Source: three-view drawing plus pictorial views. Frame: mm from the lowest corner of the part. A direction names the side the tool comes from. Give positions to 0.01 mm unless a question says otherwise; leave off trailing zeros. Order: outer loops, then holes, each group sorted by start corner. A loop starts at its lowest first (then second) coordinate and runs counter-clockwise, first axis right, second up. Notation, with made-up numbers: (57.5, -23) - (69.5, -23) arc R25 ccw to (69.5, 9) - close; hole circle Ø8 at (-7, 36). An arc over 180 degrees is marked (long way). Answer in a Markdown table with one row per item. Add a question column.
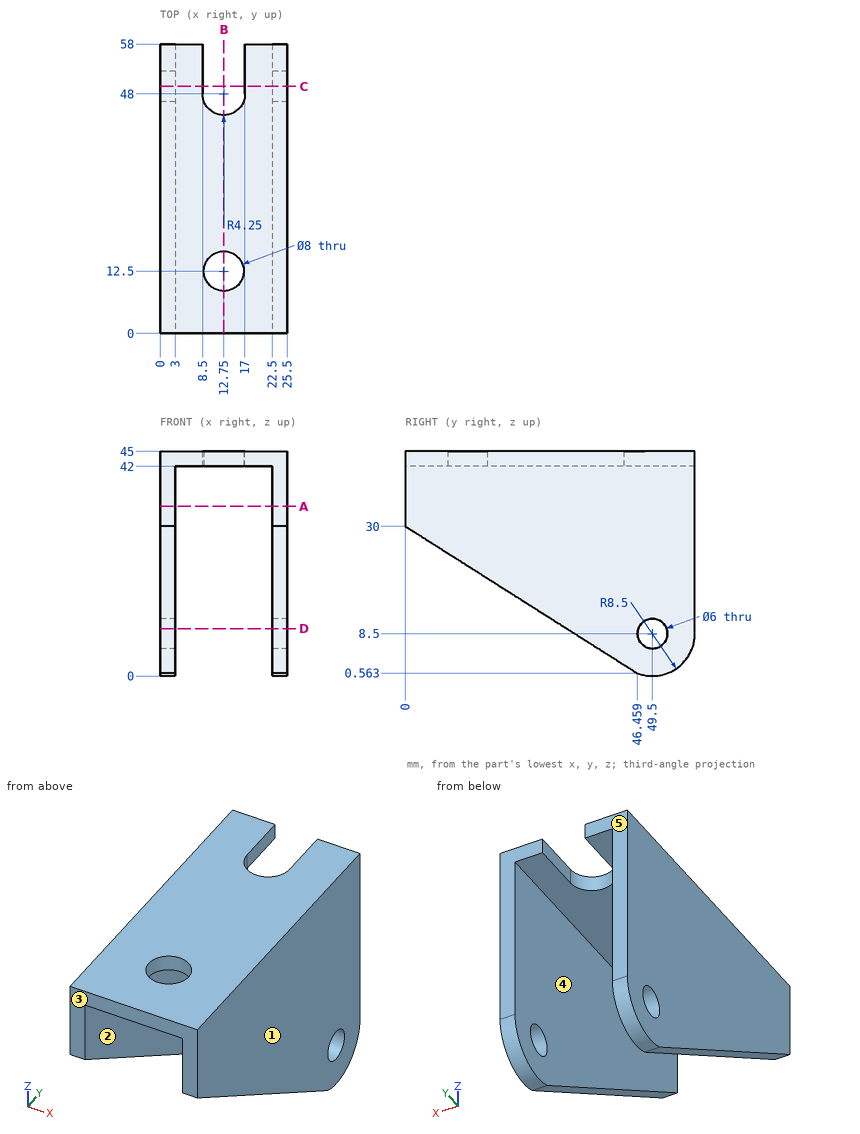
Q1. Pull-direction query (X, two-part tool) for the marked faces 1, 2 and 3; classes: +X half, -X half, draft (parallel to the pull), parting line (faces both ways), or undercut.
Q2. Section A-A, the plane z = 34. Return loops of the section in (x, y), then the cut area to 3 significant figures.
Q3. Contact query for flat-ended pins moving along their axis: P1, Ø2, axis at x = 21, z = 37.5, coming from the +Y side; P2, Ø2, axis at x = 20, y = 21, coming from the -Z side. Output: stop coordinate, or through.
Q4. Section B-B, the plane x = 12.75. Return loops of the section in (y, z).
Q5. Access query for the marked faces 4 and 5. Directions: +Z, -Z, +X, -X, +Y, -Y. A direction counts if a zero-diameter tool reaches every point of the face in a straight line with its end or side. Return the directions, or none.
Q6. Section C-C, the plane y = 49.5. Return loops of the section in (x, z), then the cut area to 3 significant figures.
Q7. Line query: probe 1 along X at (y, z) = (41, 36.5); probe 2 along Z at (x, y) = (1.15, 49.5); probe 3 along Z at (x, y) = (7.75, 49.5). Output: solid intervals per line, ascending.
Q8. Section D-D, the plane z = 9.5. Return loops of the section in (x, y).
Computed:
| question | item | result |
|---|---|---|
| 1 | face 1 | +X half |
| 1 | face 2 | undercut |
| 1 | face 3 | draft |
| 2 | outline | (0, 0) - (3, 0) - (3, 58) - (0, 58) - close; (22.5, 0) - (25.5, 0) - (25.5, 58) - (22.5, 58) - close |
| 2 | area | 348 mm^2 |
| 3 | P1 | passes through |
| 3 | P2 | stops at z = 42 |
| 4 | outline | (0, 42) - (8.5, 42) - (8.5, 45) - (0, 45) - close; (16.5, 42) - (43.75, 42) - (43.75, 45) - (16.5, 45) - close |
| 5 | face 4 | -Z, +Y, -Y |
| 5 | face 5 | +Z, -Z, +X, -X, +Y |
| 6 | outline | (0, 0) - (3, 0) - (3, 5.5) - (0, 5.5) - close; (0, 11.5) - (3, 11.5) - (3, 42) - (8.5, 42) - (8.5, 45) - (0, 45) - close; (17, 42) - (22.5, 42) - (22.5, 11.5) - (25.5, 11.5) - (25.5, 45) - (17, 45) - close; (22.5, 0) - (25.5, 0) - (25.5, 5.5) - (22.5, 5.5) - close |
| 6 | area | 267 mm^2 |
| 7 | probe 1 | x = 0 to 3, 22.5 to 25.5 |
| 7 | probe 2 | z = 0 to 5.5, 11.5 to 45 |
| 7 | probe 3 | z = 42 to 45 |
| 8 | outline | (0, 32.35) - (3, 32.35) - (3, 46.67) - (0, 46.67) - close; (0, 52.33) - (3, 52.33) - (3, 58) - (0, 58) - close; (22.5, 32.35) - (25.5, 32.35) - (25.5, 46.67) - (22.5, 46.67) - close; (22.5, 52.33) - (25.5, 52.33) - (25.5, 58) - (22.5, 58) - close |
